Part model, mm, in its own coordinate system. Face numbers are marked on the shaded views. A direction names the side the tool comes from. Give positions to 0.01 mm unless a question says otherwise; leave off trailing zeros. Order: outer loops, then holes, each group sorted by start corner. A loop starts at its lowest first (then second) coordinate and runs counter-clockwise, first axis right, second up.
1. Which spindle directions (+Z, -Z, +X, -X, +Y, -Y) get a long thin tool onto all of the face, cutting with end or side? Do the marked faces 4 and 5. Say none if no direction does.
2. Slice it at D-D on x = 47.5. List the corners of the cut face in (y, z), and give its area (3 significant figures).
3. Mould opens along X. For the marked faces 1, 2 and 3 say: +X half, -X half, draft (parallel to the pull), parting line (faces both ways), or undercut.
4. Slice it at B-B on x = 90. List the corners of the cut face in (y, z), and give its area (3 significant figures).
5. Slice it at A-A on y = -14. List the corners of the cut face in (x, z), and give its area (3 significant figures).
6. Slice it at C-C on z = 10. Give the number of separate pieces and of enclosed holes in the cut face, and give its area (3 significant figures).
7. Drop flat-ended pins along their axis: pin 1 Ø5 at (x, z) = (-91, 11.5) entering from -Y; pin 2 Ø1 at (x, z) = (20.5, 2.5) entering from +Y; pin 3 Ø5 at (x, z) = (91, 9.5) entering from -Y. Give the stop position or say it passes through.
8. Probe line 1 (X direction, y = 1.7, z = 10); line 2 (X direction, y = -3.45, z = 10); line 3 (Z direction, x = -90, y = 3.9). List the from-to ranges inside material, lowest first.
from build123d import *

# Parameters (mm, degrees)
F0_W     = 20
F0_H     = 10
F0_W_2   = 10
F1_DEPTH = 20
F3_D     = 7
F4_D     = 12
F4_DEPTH = 4
F4_TIP   = 3.6051637142
F5_R     = 5
F6_R     = 4
F7_R     = 5


with BuildPart() as f1:
    # F0 (on Top) → F1 (new body)
    with BuildSketch(Plane.XY):
        with Locations((-90, 0)):
            Rectangle(F0_W, F0_H)
        Polygon((-70, -5), (-80, -5), (-70, -33.2842712475), (70, -33.2842712475), (80, -5), (70, -5), (65, -24.6240172096), (-65, -24.6240172096), align=None)
        with Locations((-75, 0)):
            Rectangle(F0_W_2, F0_H)
        with Locations((75, 0)):
            Rectangle(F0_W_2, F0_H)
        with Locations((90, 0)):
            Rectangle(F0_W, F0_H)
    extrude(amount=F1_DEPTH)

    # F3 (through all)
    with Locations(Plane.XZ.offset(5)):
        with Locations((-90, 10), (90, 10)):
            Hole(F3_D / 2)

    # F4
    with Locations(Plane.XZ.offset(5)):
        with Locations((-90, 10), (90, 10)):
            Hole(F4_D / 2, depth=F4_DEPTH)
            with Locations((0, 0, -(F4_DEPTH + F4_TIP / 2))):  # 118° drill point
                Cone(0, F4_D / 2, F4_TIP, mode=Mode.SUBTRACT)

    # F5
    f5_edges = [f1.edges().sort_by_distance(p)[0] for p in [
        (-100, 0, 20),
        (-100, 0, 0),
        (100, 0, 20),
        (100, 0, 0),
    ]]
    fillet(f5_edges, radius=F5_R)

    # F6
    f6_edges = [f1.edges().sort_by_distance(p)[0] for p in [
        (-80, -5, 10),
        (80, -5, 10),
    ]]
    fillet(f6_edges, radius=F6_R)

    # F7
    f7_edges = [f1.edges().sort_by_distance(p)[0] for p in [
        (-70, -33.284271, 10),
        (70, -33.284271, 10),
        (-65, -24.624017, 10),
        (65, -24.624017, 10),
    ]]
    fillet(f7_edges, radius=F7_R)


solid = f1.part
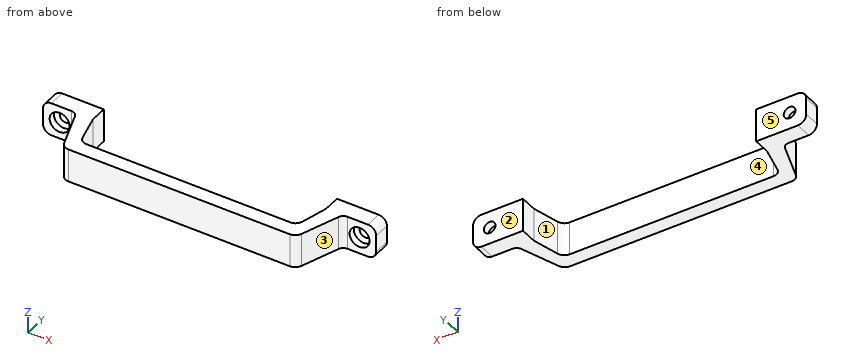
Data:
1. face 4: +Z, -Z, +Y
1. face 5: +Z, -Z, +X, -X, +Y
2. outline: (-33.28, 0) - (-24.62, 0) - (-24.62, 20) - (-33.28, 20) - close
2. area: 173 mm2
3. face 1: undercut
3. face 2: draft
3. face 3: +X half
4. outline: (-5, 0) - (5, 0) - (5, 6.5) - (0.5, 6.5) - (-1, 4) - (-5, 4) - close; (-5, 16) - (-1, 16) - (0.5, 13.5) - (5, 13.5) - (5, 20) - (-5, 20) - close
4. area: 106 mm2
5. outline: (-76.82, 0) - (-67.71, 0) - (-67.71, 20) - (-76.82, 20) - close; (67.71, 0) - (76.82, 0) - (76.82, 20) - (67.71, 20) - close
5. area: 364 mm2
6. separate pieces: 3
6. enclosed holes: 0
6. area: 2,010 mm2
7. pin 1: stops at y = 0.02
7. pin 2: stops at y = -24.62
7. pin 3: stops at y = 0.43
8. line 1: x = -100 to -93.5, -86.5 to -70, 70 to 86.5, 93.5 to 100
8. line 2: x = -100 to -96, -84 to -70, 70 to 84, 96 to 100
8. line 3: z = 0 to 6.5, 13.5 to 20
